```python
from build123d import *

# Parameters (mm, degrees)
SKETCH2_R           = 50.8
SKETCH2_R_2         = 8.255
BOSS_EXTRUDE2_DEPTH = 9.525


with BuildPart() as part:
    # Sketch2 → Boss-Extrude2 (new body)
    with BuildSketch(Plane.XY):
        with Locations(Location((0, 0, 0), (0, 0, 180))):
            Circle(SKETCH2_R)
        with Locations(Location((-28.284214679, 28.284214679, 0), (0, 0, 180))):
            Circle(SKETCH2_R_2, mode=Mode.SUBTRACT)
        with Locations(Location((28.284214679, 28.284214679, 0), (0, 0, 180))):
            Circle(SKETCH2_R_2, mode=Mode.SUBTRACT)
        with Locations(Location((28.284214679, -28.284214679, 0), (0, 0, 180))):
            Circle(SKETCH2_R_2, mode=Mode.SUBTRACT)
        with Locations(Location((-28.284214679, -28.284214679, 0), (0, 0, 180))):
            Circle(SKETCH2_R_2, mode=Mode.SUBTRACT)
    extrude(amount=BOSS_EXTRUDE2_DEPTH)


solid = part.part
```
Input: part model. Units: mm. Frame: model coordinates. Round coordinates to 2 decimals unless told otherwise and drop trailing zeros. Order: outer loops, then holes, each group sorted by start corner. A loop starts at its lowest first (then second) coordinate and runs counter-clockwise, first axis right, second up. Notation, with made-up numbers: (2.25, 18) - (39.25, 18) arc R38 ccw to (39.25, 57) - close; hole circle Ø5 at (-18, 25.5). An arc over 180 degrees is marked (long way). One line per question, with ' | ' between items. Start each with the question number.
1) Cut plane C-C, the plane z = 1.25. Return the cut outline in (x, y) (3 decimals).
2) Contact query for flat-ended pins moving along their axis: P1, Ø1.5, axis at y = 29.5, z = 2, coming from the -X side; P2, Ø1.5, axis at x = 33, y = -32.5, coming from the -Z side; P3, Ø5, axis at y = -28, z = 3, coming from the -X side; P4, Ø1, axis at y = -36, z = 3.5, coming from the +X side. Output: stop coordinate, or through.
3) Cut plane D-D, the plane x = -9. Return the cut outline in (y, z) (3 decimals), then the cut area to 3 significant figures.
4) Cut plane A-A, the plane y = 33. Return the cut outline in (x, z) (3 decimals).
5) Cut plane B-B, the plane x = -33.5. Return the cut outline in (y, z) (3 decimals), then the cut area to 3 significant figures.
6) Pull-direction query (X, two-part tool) for faces 1 (the cylindrical face through (-23.44, 45.07, 4.7)), 2 (the flat face through (1, -1, 0)), 3 (the cylindrical face through (-32.722, -35.245, 4.696)); classes: +X half, -X half, draft (parallel to the pull), parting line (faces both ways), or undercut.
7) Ray query, probe 1 along X at (y, z) = (32, 7.5); probe 2 along Y at (x, z) = (22.5, 8.5); probe 3 along Y at (x, z) = (22, 8). Return the intervals inside material, ascending.
Worked out:
1) outline: circle Ø101.6 at (0, 0); hole circle Ø16.51 at (-28.284, -28.284); hole circle Ø16.51 at (-28.284, 28.284); hole circle Ø16.51 at (28.284, -28.284); hole circle Ø16.51 at (28.284, 28.284)
2) P1: stops at x = -41.88 | P2: passes through | P3: stops at x = -43.94 | P4: stops at x = 36.34
3) outline: (-49.996, 0) - (49.996, 0) - (49.996, 9.525) - (-49.996, 9.525) - close | area: 952 mm^2
4) outline: (-38.622, 0) - (-35.06, 0) - (-35.06, 9.525) - (-38.622, 9.525) - close; (-21.509, 0) - (21.509, 0) - (21.509, 9.525) - (-21.509, 9.525) - close; (35.06, 0) - (38.622, 0) - (38.622, 9.525) - (35.06, 9.525) - close
5) outline: (-38.189, 0) - (-34.683, 0) - (-34.683, 9.525) - (-38.189, 9.525) - close; (-21.886, 0) - (21.886, 0) - (21.886, 9.525) - (-21.886, 9.525) - close; (34.683, 0) - (38.189, 0) - (38.189, 9.525) - (34.683, 9.525) - close | area: 484 mm^2
6) face 1: parting line | face 2: draft | face 3: undercut
7) probe 1: x = -39.45 to -35.66, -20.91 to 20.91, 35.66 to 39.45 | probe 2: y = -45.55 to -34.17, -22.39 to 22.39, 34.17 to 45.55 | probe 3: y = -45.79 to -33.64, -22.93 to 22.93, 33.64 to 45.79
